Could you check a few things on this model? Use its own coordinates, in mm. Face numbers are marked on the shaded views. A direction names the side the tool comes from. Round coordinates to 2 decimals unless told otherwise and drop trailing zeros. Write each loop counter-clockwise with the first axis right and the second up, starting at its lowest first coordinate (ties: lowest second). Pieces come first, ordered by that corner, then holes. Notation, with made-up numbers: (-2.5, 59) - (19.5, 59) arc R6 ccw to (19.5, 69) - close; hole circle Ø1 at (12.25, 3.25). An arc over 180 degrees is marked (long way). Put each result on its own line as item: value.
Autodesk Inventor part; units mm, degrees
ref_plane "YZ Plane" through (0, 0, 0) normal (1, 0, 0) x (0, 1, 0)
ref_plane "XZ Plane" through (0, 0, 0) normal (0, 1, 0) x (-1, 0, 0)
ref_plane "XY Plane" through (0, 0, 0) normal (0, 0, 1) x (1, 0, 0)
sketch "Esquisse1" plane through (0, 0, 0) normal (0, 0, 1) x (1, 0, 0)
  line L0 (-6, 11.6) -> (6, 11.6) construction
  line L1 (6, 11.6) -> (6, -11.6) construction
  line L2 (6, -11.6) -> (-6, -11.6) construction
  line L3 (-6, -11.6) -> (-6, 11.6) construction
  line L4 (-6, 11.6) -> (6, -11.6) construction
  line L5 (-6, -11.6) -> (6, 11.6) construction
  line L6 (-3.7, -11.6) -> (3.7, -11.6)
  line L7 (3.7, -11.6) -> (3.7, -13.6)
  line L8 (-3.7, -13.6) -> (-3.7, -11.6)
  line L9 (-5.75, -19.6) -> (6.25, -19.6)
  line L10 (-5.75, -13.6) -> (-5.75, -19.6)
  line L11 (5.75, -13.6) -> (3.7, -13.6)
  line L12 (-3.7, -13.6) -> (-5.75, -13.6)
  circle A0 centre (0, -14) radius 1.6
  line L13 (-3.7, -13.6) -> (0, -14) construction
  line L14 (0, -14) -> (3.7, -13.6) construction
  line L15 (-6, 0) -> (6, 0) construction
  line L16 (6, 0) -> (28.3304, 0) construction
  line L17 (7.75, 0) -> (7.75, -13.6)
  line L18 (12.25, -19.6) -> (12.25, 0)
  line L19 (5.75, -13.6) -> (7.75, -13.6)
  line L20 (6.25, -19.6) -> (12.25, -19.6)
  line L21 (6, -11.6) -> (6, 11.6) construction
  line L22 (6, 11.6) -> (-6, 11.6) construction
  line L23 (-6, 11.6) -> (-6, -11.6) construction
  line L24 (-6, -11.6) -> (6, 11.6) construction
  line L25 (-6, 11.6) -> (6, -11.6) construction
  line L26 (-3.7, 11.6) -> (3.7, 11.6)
  line L27 (3.7, 11.6) -> (3.7, 13.6)
  line L28 (-3.7, 13.6) -> (-3.7, 11.6)
  line L29 (-5.75, 19.6) -> (6.25, 19.6)
  line L30 (-5.75, 13.6) -> (-5.75, 19.6)
  line L31 (5.75, 13.6) -> (3.7, 13.6)
  line L32 (-3.7, 13.6) -> (-5.75, 13.6)
  circle A1 centre (0, 14) radius 1.6
  line L33 (-3.7, 13.6) -> (0, 14) construction
  line L34 (0, 14) -> (3.7, 13.6) construction
  line L35 (7.75, 0) -> (7.75, 13.6)
  line L36 (12.25, 19.6) -> (12.25, 0)
  line L37 (5.75, 13.6) -> (7.75, 13.6)
  line L38 (6.25, 19.6) -> (12.25, 19.6)
  point P0 (0, 0)
  point P1 (0, 0)
  point P2 (0, -11.6)
  point P3 (0, 11.6)
  dimension "d0" = 23.2
  dimension "d1" = 12
  dimension "d2" = 7.4
  dimension "d4" = 2
  dimension "d6" = 2.4
  dimension "d7" = 3.2
  dimension "d8" = 6
  dimension "d9" = 18
  dimension "d10" = 2
  dimension "d11" = 4.5
extrude "Extrusion1" add sketch "Esquisse1" along normal blind 5
sketch "Esquisse2" plane through (0, 0, 5) normal (0, 0, 1) x (1, 0, 0)
  circle A0 centre (0, 14) radius 1.6 construction
  line L0 (12.25, -19.6) -> (12.25, 19.6) construction
  line L1 (3.7, -13.6) -> (3.7, -11.6) construction
  circle A1 centre (0, 14) radius 3.75
  line L2 (12.25, 0) -> (-17.9145, 0) construction
  circle A2 centre (0, -14) radius 3.75
  point P0 (0, 0)
  dimension "d14" = 7.5
extrude "Extrusion2" cut sketch "Esquisse2" against normal blind 3
fillet "Congé1" radius 1 4 edges at (3.7, 11.6, 2.5) (-3.7, 11.6, 2.5) (3.7, -11.6, 2.5) (-3.7, -11.6, 2.5)
fillet "Congé2" radius 1 4 edges at (-5.75, 13.6, 2.5) (-5.75, 19.6, 2.5) (-5.75, -13.6, 2.5) (-5.75, -19.6, 2.5)
properties part number "FixationCorona"
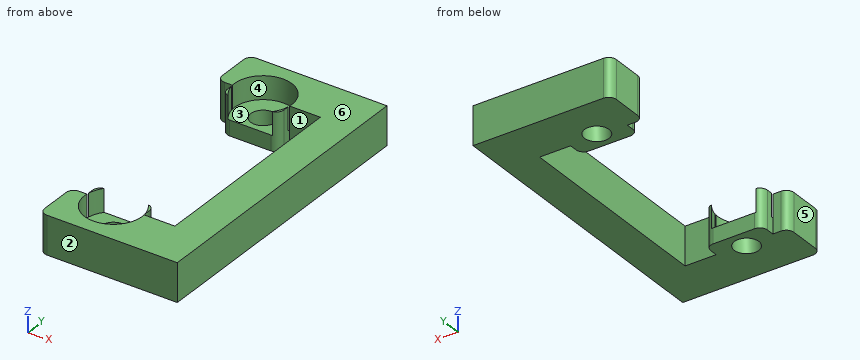
(1) Imagine slicing it at B-B, the plane z = 1.35. List the corners of the cut face in (x, y) for me.
Values found:
outline: (-5.75, -18.6) arc R1 ccw to (-4.75, -19.6) - (12.25, -19.6) - (12.25, 19.6) - (-4.75, 19.6) arc R1 ccw to (-5.75, 18.6) - (-5.75, 14.6) arc R1 ccw to (-4.75, 13.6) - (-3.7, 13.6) - (-3.7, 12.6) arc R1 ccw to (-2.7, 11.6) - (2.7, 11.6) arc R1 ccw to (3.7, 12.6) - (3.7, 13.6) - (7.75, 13.6) - (7.75, -13.6) - (3.7, -13.6) - (3.7, -12.6) arc R1 ccw to (2.7, -11.6) - (-2.7, -11.6) arc R1 ccw to (-3.7, -12.6) - (-3.7, -13.6) - (-4.75, -13.6) arc R1 ccw to (-5.75, -14.6) - close; hole circle Ø3.2 at (0, -14); hole circle Ø3.2 at (0, 14)
(2) I'm going to push flat-ended pins straight in: pin 1 (8 mm diameter, centred on x = 3, y = 0, fed in from -Z); pin 2 (0.8 mm diameter, centred on y = -13, z = 2, fed in from -X); pin 3 (3.5 mm diameter, centred on x = 0, y = 14, fed in from +Z). Where does each tip first touch, or does it pass through?
Values found:
pin 1: passes through
pin 2: stops at x = -3.7
pin 3: stops at z = 2
(3) For the marked faces 1, 2 and 3, which set-ups out of +Z, -Z, +X, -X, +Y, -Y let a thin tool reach every point of the face, with its end or its side?
Values found:
face 1: +Z, -Z
face 2: +Z, -Z, +X, -X, -Y
face 3: +Z
(4) Imagine slicing it at C-C, the plane x = 0. List the corners of the cut face in (y, z) for me, then the cut area to 3 significant figures.
Values found:
outline: (-19.6, 0) - (-15.6, 0) - (-15.6, 2) - (-17.75, 2) - (-17.75, 5) - (-19.6, 5) - close; (-12.4, 0) - (-11.6, 0) - (-11.6, 2) - (-12.4, 2) - close; (11.6, 0) - (12.4, 0) - (12.4, 2) - (11.6, 2) - close; (15.6, 0) - (19.6, 0) - (19.6, 5) - (17.75, 5) - (17.75, 2) - (15.6, 2) - close
area: 30.3 mm^2
(5) Imagine slicing it at D-D, the plane z = 4. List the corners of the cut face in (x, y) for me, then the cut area to 3 significant figures.
Values found:
outline: (-5.75, -18.6) arc R1 ccw to (-4.75, -19.6) - (12.25, -19.6) - (12.25, 19.6) - (-4.75, 19.6) arc R1 ccw to (-5.75, 18.6) - (-5.75, 14.6) arc R1 ccw to (-4.75, 13.6) - (-3.73, 13.6) arc R3.75 cw (long way) to (3.73, 13.6) - (7.75, 13.6) - (7.75, -13.6) - (3.73, -13.6) arc R3.75 cw (long way) to (-3.73, -13.6) - (-4.75, -13.6) arc R1 ccw to (-5.75, -14.6) - close; (-3.7, -13.39) arc R3.75 cw to (-2.9, -11.62) arc R1 ccw to (-3.7, -12.6) - close; (-3.7, 12.6) arc R1 ccw to (-2.9, 11.62) arc R3.75 cw to (-3.7, 13.39) - close; (2.9, -11.62) arc R3.75 cw to (3.7, -13.39) - (3.7, -12.6) arc R1 ccw to start; (2.9, 11.62) arc R1 ccw to (3.7, 12.6) - (3.7, 13.39) arc R3.75 cw to start
area: 289 mm^2
(6) If we mould it in two halves opening along X, with no side actions, what happens to the marked faces 4, 5 and 6? For each: pulls with the +X half, pulls with the -X half, needs draft (parallel to the pull), parting line crosses it, or undercut.
Values found:
face 4: undercut
face 5: pulls with the -X half
face 6: needs draft
(7) Imagine slicing it at A-A, the plane y = -14. List the corners of the cut face in (x, z) for me, then the cut area to 3 significant figures.
Values found:
outline: (-5.55, 0) - (-1.6, 0) - (-1.6, 2) - (-3.75, 2) - (-3.75, 5) - (-5.55, 5) - close; (1.6, 0) - (12.25, 0) - (12.25, 5) - (3.75, 5) - (3.75, 2) - (1.6, 2) - close
area: 60.1 mm^2
(8) Please list where these lines run through material, in increasing order: probe 1 along Y at (x, z) = (0, 0.55); probe 2 along Y at (x, z) = (6.25, 3.7); probe 3 along Y at (x, z) = (0, 4.15). Write a range as from..to.
Values found:
probe 1: y = -19.6..-15.6, -12.4..-11.6, 11.6..12.4, 15.6..19.6
probe 2: y = -19.6..-13.6, 13.6..19.6
probe 3: y = -19.6..-17.75, 17.75..19.6
